Source: CAD feature listing. Evaluate the final solid. Frame: model axes, mm. Face numbers are marked on the shaded views. Coordinates: 2 decimals unless noted, no trailing zeros. Order: outer loops, then holes, each group sorted by start corner. A loop starts at its lowest first (then second) coordinate and runs counter-clockwise, first axis right, second up.
```python
from build123d import *

# Parameters (mm, degrees)
F0_W     = 12.7
F0_H     = 25.4
F0_R     = 1.014077
F0_R_2   = 0.9525
F1_DEPTH = 3.175
F3_DEPTH = 12.7


with BuildPart() as f1:
    # F0 (on Right) → F1 (new body)
    with BuildSketch(Plane.YZ):
        with Locations((-6.35, 12.7)):
            Rectangle(F0_W, F0_H)
        with Locations((-9.525, 22.86)):
            Circle(F0_R, mode=Mode.SUBTRACT)
        with Locations((-3.175, 22.86)):
            Circle(F0_R_2, mode=Mode.SUBTRACT)
    extrude(amount=F1_DEPTH)

    # F2 (on Top) → F3 (join)
    with BuildSketch(Plane.XY):
        with BuildLine():
            ThreePointArc((5.334, -8.509), (3.807356, -7.876644), (3.175, -6.35))
            Line((3.175, -6.35), (3.175, -12.664954))
            Line((3.175, -12.664954), (5.334, -8.509))
        make_face()
        with BuildLine():
            ThreePointArc((3.175, -6.35), (3.807356, -4.823356), (5.334, -4.191))
            Line((5.334, -4.191), (3.175, 0))
            Line((3.175, 0), (3.175, -6.35))
        make_face()
    extrude(amount=F3_DEPTH)


solid = f1.part
```
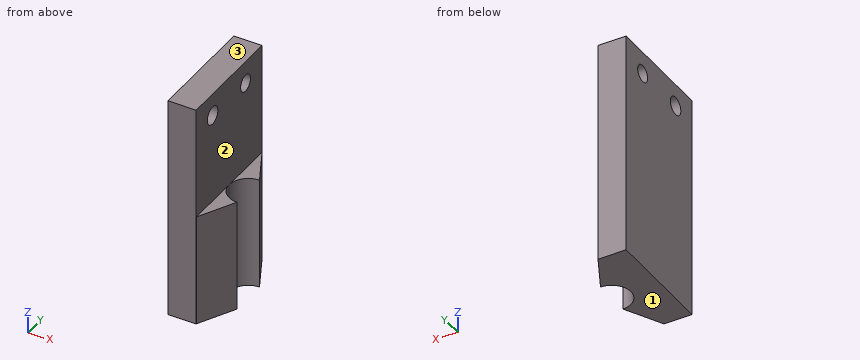
Q1. Section query C-C on y = -3. Output: boundary loops of the cut face in (x, z) (3 decimals).
Solutions:
outline: (0, 0) - (4.72, 0) - (4.72, 12.7) - (3.175, 12.7) - (3.175, 21.924) - (0, 21.924) - close; (0, 23.796) - (3.175, 23.796) - (3.175, 25.4) - (0, 25.4) - close
Q2. Pull-direction query (Z, two-part tool) for the marked faces 1, 2 and 3; classes: pulls with the +Z half, pulls with the -Z half, needs draft (parallel to the pull), parting line crosses it, or undercut.
Solutions:
face 1: pulls with the -Z half
face 2: needs draft
face 3: pulls with the +Z half
Q3. Material intervals for line 1 along X through (y, z) = (-6.5, 23.25) (3 decimals); line 2 along Y through (x, z) = (3.9, 3.25); line 3 along Z through (x, y) = (2, -3.5), sorted ascending.
Solutions:
line 1: x = 0 to 3.175
line 2: y = -11.27 to -7.96, -4.74 to -1.41
line 3: z = 0 to 21.96, 23.76 to 25.4
Q4. Pin query (flat end, axial travel): P1, Ø3, axis at y = -6, z = 3, coming from the +X side; P2, Ø2, axis at x = 4.5, y = -10.5, coming from the +Z side; P3, Ø2, axis at y = -3, z = 5.5, coming from the +X side. Return the tip coordinate at first contact, or that it passes through.
Solutions:
P1: stops at x = 4.22
P2: stops at z = 12.7
P3: stops at x = 5.24
Q5. Section query D-D on x = 1.8. Output: boundary loops of the cut face in (y, z) (1 decimal).
Solutions:
outline: (-12.7, 0) - (0, 0) - (0, 25.4) - (-12.7, 25.4) - close; hole circle Ø2 at (-9.5, 22.9); hole circle Ø1.9 at (-3.2, 22.9)
Q6. Section query A-A on z = 22.86. Output: boundary loops of the cut face in (x, y) (1 decimal), plus the area to 3 significant figures.
Solutions:
outline: (0, -12.7) - (3.2, -12.7) - (3.2, -10.5) - (0, -10.5) - close; (0, -8.5) - (3.2, -8.5) - (3.2, -4.1) - (0, -4.1) - close; (0, -2.2) - (3.2, -2.2) - (3.2, 0) - (0, 0) - close
area: 27.8 mm2
Q7. Section query B-B on z = 3. Output: boundary loops of the cut face in (x, y) (3 decimals), plus the area to 3 significant figures.
Solutions:
outline: (0, -12.7) - (3.175, -12.7) - (3.175, -12.665) - (5.334, -8.509) arc R2.159 cw to (3.175, -6.35) arc R2.159 cw to (5.334, -4.191) - (3.175, 0) - (0, 0) - close
area: 51.3 mm2
